Model file for the job. Use its own axes, mm. Coordinates: 2 decimals unless noted, no trailing zeros. Loops run counter-clockwise (first coordinate to the right, second up) from the corner with the lowest first, then second, coordinate; pieces in that order, holes last.
from build123d import *

# Parameters (mm, degrees)
F1_R     = 9
F2_DEPTH = 7
F3_R     = 0.5
F4_R     = 0.3
F5_R     = 0.3
F6_R     = 0.3


with BuildPart() as f2:
    # F1 (on Top) → F2 (new body)
    with BuildSketch(Plane.XY):
        Polygon((4.4527957955, 10.75), (-4.4527957955, 10.75), (-10.75, 4.4527957955), (-10.75, -4.4527957955), (-4.4527957955, -10.75), (4.4527957955, -10.75), (10.75, -4.4527957955), (10.75, 4.4527957955), align=None)
        Circle(F1_R, mode=Mode.SUBTRACT)
    extrude(amount=F2_DEPTH)

    # F3
    f3_edges = [f2.edges().sort_by_distance(p)[0] for p in [
        (7.601398, 7.601398, 7),
        (0, 10.75, 7),
        (-7.601398, 7.601398, 7),
        (-10.75, 0, 7),
        (-7.601398, -7.601398, 7),
        (0, -10.75, 7),
        (7.601398, -7.601398, 7),
        (10.75, 0, 7),
    ]]
    fillet(f3_edges, radius=F3_R)

    # F4
    f4_edges = [f2.edges().sort_by_distance(p)[0] for p in [
        (0, -10.75, 0),
        (-7.601398, -7.601398, 0),
        (-10.75, 0, 0),
        (-7.601398, 7.601398, 0),
        (0, 10.75, 0),
        (7.601398, 7.601398, 0),
        (10.75, 0, 0),
        (7.601398, -7.601398, 0),
    ]]
    fillet(f4_edges, radius=F4_R)

    # F5
    f5_edges = [f2.edges().sort_by_distance(p)[0] for p in [
        (-9, 0, 0),
    ]]
    fillet(f5_edges, radius=F5_R)

    # F6
    f6_edges = [f2.edges().sort_by_distance(p)[0] for p in [
        (-9, 0, 7),
    ]]
    fillet(f6_edges, radius=F6_R)


solid = f2.part
Q1. Slice it at B-B (y = 0). List the corners of the cut face in (x, z).
Answers:
outline: (-10.75, 0.3) arc R0.3 ccw to (-10.45, 0) - (-9.3, 0) arc R0.3 ccw to (-9, 0.3) - (-9, 6.7) arc R0.3 ccw to (-9.3, 7) - (-10.25, 7) arc R0.5 ccw to (-10.75, 6.5) - close; (9, 0.3) arc R0.3 ccw to (9.3, 0) - (10.45, 0) arc R0.3 ccw to (10.75, 0.3) - (10.75, 6.5) arc R0.5 ccw to (10.25, 7) - (9.3, 7) arc R0.3 ccw to (9, 6.7) - close
Q2. Flat gauge pin, fed straight in: P1, Ø1.5, axis at x = -5.5, z = 3, coming from the +Y side. Where does the tip first touch, or does it go through?
Answers:
P1: stops at y = 10.45
Q3. Mould opens along X. For faces 1 (the cylindrical face through (7.46, 7.54, 6.85)), 2 (the flat face through (-7.6, 7.6, 3.4)), 3 (the cylindrical face through (-1.172, 8.923, 3.455)) say: +X half, -X half, draft (parallel to the pull), parting line (faces both ways), or undercut.
Answers:
face 1: +X half
face 2: -X half
face 3: undercut
Q4. Drill centre lines: line 1 (Y direction, x = 0, z = 4.25); line 2 (X direction, y = 1.25, z = 3); line 3 (Y direction, x = -2.5, z = 3.75). Where is each one in solid material? Low to high.
Answers:
line 1: y = -10.75 to -9, 9 to 10.75
line 2: x = -10.75 to -8.91, 8.91 to 10.75
line 3: y = -10.75 to -8.65, 8.65 to 10.75
Q5. Slice it at A-A (z = 2.25). List the corners of the cut face in (x, y), and give its area (3 significant figures).
Answers:
outline: (-10.75, -4.45) - (-4.45, -10.75) - (4.45, -10.75) - (10.75, -4.45) - (10.75, 4.45) - (4.45, 10.75) - (-4.45, 10.75) - (-10.75, 4.45) - close; hole circle Ø18 at (0, 0)
area: 128 mm2
